from build123d import *

# Parameters (mm, degrees)
SKETCH_1_R             = 2
SM_BASE_FLANGE_1_DEPTH = 0.7
OTHER_START            = -25
OTHER_1_DEPTH          = 50
OTHER_1_2_DEPTH        = 10
OTHER_START_2          = -5
OTHER_1_3_DEPTH        = 10
OTHER_START_3          = 15
OTHER_1_4_DEPTH        = 10


# Read off the part's stored shape, not the designer's step: 褶边1
# Sheet-metal steps are written as plain solids
with BuildPart() as part:
    # Sketch 1 → 基体-法兰1 (new body)
    with BuildSketch(Plane(origin=(0, 0, 0), x_dir=(1, 0, 0), z_dir=(0, 1, 0))):
        Polygon((0, 0), (-25, 0), (-25, 18), (-15, 18), (-15, 13), (-5, 13), (-5, 18), (5, 18), (5, 13), (15, 13), (15, 18), (25, 18), (25, 0), align=None)
        with Locations(Location((-15, 5.5, 0), (0, 0, 270))):
            Circle(SKETCH_1_R, mode=Mode.SUBTRACT)
        with Locations(Location((15, 5.5, 0), (0, 0, 90))):
            Circle(SKETCH_1_R, mode=Mode.SUBTRACT)
    extrude(amount=-SM_BASE_FLANGE_1_DEPTH)

    # Other 1 outline → Other 1 (cut)
    with BuildSketch(Plane.YZ.offset(OTHER_START)):
        with BuildLine():
            Line((0, -18), (0, -17.264642819))
            ThreePointArc((0, -17.264642819), (-0.518259244, -16.476012959), (-0.7, -15.55))
            Line((-0.7, -15.55), (-0.7, -18))
            Line((-0.7, -18), (0, -18))
        make_face()
    extrude(amount=OTHER_1_DEPTH, mode=Mode.SUBTRACT)

    # Other 1 2 outline → Other 1 2 (add)
    with BuildSketch(Plane.YZ.offset(OTHER_START)):
        with BuildLine():
            Line((0.175170356, -13.673191114), (0.625121683, -14.209422225))
            ThreePointArc((0.625121683, -14.209422225), (3.336038627, -16.289581958), (0, -15.55))
            Line((0, -15.55), (0, -17.264642819))
            ThreePointArc((0, -17.264642819), (4.197091003, -15.669355023), (0.175170356, -13.673191114))
        make_face()
    extrude(amount=OTHER_1_2_DEPTH)

    # Other 1 3 outline → Other 1 3 (add)
    with BuildSketch(Plane.YZ.offset(OTHER_START_2)):
        with BuildLine():
            Line((0.175170356, -13.673191114), (0.625121683, -14.209422225))
            ThreePointArc((0.625121683, -14.209422225), (3.336038627, -16.289581958), (0, -15.55))
            Line((0, -15.55), (0, -17.264642819))
            ThreePointArc((0, -17.264642819), (4.197091003, -15.669355023), (0.175170356, -13.673191114))
        make_face()
    extrude(amount=OTHER_1_3_DEPTH)

    # Other 1 4 outline → Other 1 4 (add)
    with BuildSketch(Plane.YZ.offset(OTHER_START_3)):
        with BuildLine():
            Line((0.175170356, -13.673191114), (0.625121683, -14.209422225))
            ThreePointArc((0.625121683, -14.209422225), (3.336038627, -16.289581958), (0, -15.55))
            Line((0, -15.55), (0, -17.264642819))
            ThreePointArc((0, -17.264642819), (4.197091003, -15.669355023), (0.175170356, -13.673191114))
        make_face()
    extrude(amount=OTHER_1_4_DEPTH)


solid = part.part
CAD build for the part. Positions are in the model's coordinates, mm. A direction names the side the tool comes from. Give positions to 0.01 mm unless a question says otherwise; leave off trailing zeros. Loops run counter-clockwise (first coordinate to the right, second up) from the corner with the lowest first, then second, coordinate; pieces in that order, holes last. Notation, with made-up numbers: M -20,52 L -10,52 A34 ccw -10,84 Z; hole C -13.75,7 d8. An arc over 180 degrees is marked long. One line per question, with ' | ' between items. Start each with the question number.
1. Saw through at A-A on y = 1.75. Give the cut face in (x, z).
2. Saw through at D-D on z = -12.5. Give the cut face in (x, y).
3. Two-plate mould, pull along Y, no slides. Class faces 1 (the face through (-0.07, 3.363, -16.229)), 2 (the face through (0, -0.7, -8)), 3 (the face through (19.93, 3.363, -16.229)), 4 (the face through (-15, 0, -17)): pulls with the +Y half, pulls with the -Y half, needs draft (parallel to the pull), parting line crosses it, or undercut.
4. Saw through at B-B on z = -5.5. Give the cut face in (x, y).
5. Flat gauge pins, fed straight in: pin 1 (2.5 mm diameter, centred on y = 1.5, z = -15.5, fed in from +X); pin 2 (5 mm diameter, centred on x = -15, z = -5.5, fed in from +Y); pin 3 (0.8 mm diameter, centred on x = -8, y = 0, fed in from -Z). Where does each tip first touch, or does it go through?
6. Probe L1, parallel to X at y = 0.1, z = -16.75; L2, parallel to X at y = -0.45, z = -5.5; L3, parallel to Z at x = -17.5, y = 1.75. List the from-to ranges inside material, lowest first. Write a range as from..to.
7. Saw through at C-C on x = 19. Give the cut face in (y, z).
8. 3-axis set-ups, long thin cutter, end or side, ignore diameter. For faces 5 (the face through (25, -0.3, -11)), 6 (the face through (-5, 0, -17)): which of +Z, -Z, +X, -X, +Y, -Y reach the whole face in a straight line?
Result sheet:
1) outline: M -25,-18 L -15,-18 L -15,-17.3 L -25,-17.3 Z; M -25,-13.8 L -15,-13.8 L -15,-13.1 L -25,-13.1 Z; M -5,-18 L 5,-18 L 5,-17.3 L -5,-17.3 Z; M -5,-13.8 L 5,-13.8 L 5,-13.1 L -5,-13.1 Z; M 15,-18 L 25,-18 L 25,-17.3 L 15,-17.3 Z; M 15,-13.8 L 25,-13.8 L 25,-13.1 L 15,-13.1 Z
2) outline: M -25,-0.7 L 25,-0.7 L 25,0 L -25,0 Z
3) face 1: undercut | face 2: pulls with the -Y half | face 3: undercut | face 4: needs draft
4) outline: M -25,-0.7 L -17,-0.7 L -17,0 L -25,0 Z; M -13,-0.7 L 13,-0.7 L 13,0 L -13,0 Z; M 17,-0.7 L 25,-0.7 L 25,0 L 17,0 Z
5) pin 1: passes through | pin 2: stops at y = 0 | pin 3: stops at z = -13
6) L1: x = -25..-15, -5..5, 15..25 | L2: x = -25..-17, -13..13, 17..25 | L3: z = -18..-17.3, -13.8..-13.1
7) outline: M -0.7,-15.55 A2.45 ccw long 0.18,-13.67 L 0.63,-14.21 A1.75 cw long 0,-15.55 L 0,0 L -0.7,0 Z
8) face 5: +Z, -Z, +X, +Y, -Y | face 6: -Z, +Y, -Y
